Here's how the part is built. I have some questions about the finished solid (model axes, mm). A direction names the side the tool comes from. Coordinates: 2 decimals unless noted, no trailing zeros. Write each loop counter-clockwise with the first axis right and the second up, starting at its lowest first coordinate (ties: lowest second). Pieces come first, ordered by that corner, then holes.
(1) Which directions (+Z, -Z, +X, -X, +Y, -Y) give clear straight access to the entire face, cutting with the end or side of a thin tool? Please do faces 4 (the flat face through (30, 29, 11)), 5 (the flat face through (-30, 29, 11)), 6 (the flat face through (40, 17, 0)), 7 (the cylindrical face through (23.846, 22.675, -7.509)).
(2) Imagine slicing it at B-B, the plane y = 24. List the corners of the cut face in (x, z) for me, plus the area to 3 significant figures.
(3) Please list where these lines run through material, in increasing order: probe 1 along X at (y, z) = (27, 0); probe 2 along X at (y, z) = (4.5, 0); probe 3 along Z at (x, y) = (35.5, 30.5).
(4) Imagine slicing it at C-C, the plane x = 6. List the corners of the cut face in (y, z) for me.
(5) Imagine slicing it at A-A, the plane z = 0. List the corners of the cut face in (x, y) for me, plus the area to 3 significant figures.
(6) For pin 1 Ø10 at (x, y) = (-10.5, 8) entering from -Z; pin 2 Ø3 at (x, y) = (13, 24) entering from +Z; pin 3 Ø3 at (y, z) = (16.5, 26) entering from +X, each with a flat end and sliding along its axis, tell me the tip position at first contact or that it passes through.
(7) Imagine slicing it at D-D, the plane y = 7.5. List the corners of the cut face in (x, z) for me.
(8) Thinking about a two-plate mould opening in X: for faces 1 (the cylindrical face through (-0.37, 5.07, 10.65)), 2 (the flat face through (-30, 29, -12)), 3 (the flat face through (30, 6, 11)), which applies, released by +X, released by -X, zero draft, split by the parting line, or undercut?
```python
from build123d import *

# Parameters (mm, degrees)
BOSS_EXTRUDE1_DEPTH = 35
SKETCH2_R           = 2.8
CUT_EXTRUDE1_DEPTH  = 10
CUT_EXTRUDE2_START  = -80
SKETCH2_2_R         = 2.8
CUT_EXTRUDE2_DEPTH  = 10
SKETCH3_R           = 1.69
SKETCH3_R_2         = 2.25
CUT_EXTRUDE3_DEPTH  = 36
SKETCH4_R           = 25
CUT_EXTRUDE4_DEPTH  = 25


with BuildPart() as part:
    # Sketch1 → Boss-Extrude1 (new body)
    with BuildSketch(Plane(origin=(0, 0, 0), x_dir=(1, 0, 0), z_dir=(0, 1, 0))):
        with BuildLine():
            Line((-40, 17.5), (-40, -17.5))
            ThreePointArc((-40, -17.5), (0, -43.660622991), (40, -17.5))
            Line((40, -17.5), (40, 17.5))
            ThreePointArc((40, 17.5), (0, 43.660622991), (-40, 17.5))
        make_face()
    extrude(amount=BOSS_EXTRUDE1_DEPTH)

    # Sketch2 → Cut-Extrude1 (cut)
    with BuildSketch(Plane.ZY.offset(40)):
        with Locations((-11.5, 29)):
            Circle(SKETCH2_R)
        with Locations((11.5, 29)):
            Circle(SKETCH2_R)
        with Locations((-11.5, 6)):
            Circle(SKETCH2_R)
        with Locations((11.5, 6)):
            Circle(SKETCH2_R)
    extrude(amount=-CUT_EXTRUDE1_DEPTH, mode=Mode.SUBTRACT)

    # Sketch2<2> → Cut-Extrude2 (cut)
    with BuildSketch(Plane.ZY.offset(40).offset(CUT_EXTRUDE2_START)):
        with Locations((-11.5, 29)):
            Circle(SKETCH2_2_R)
        with Locations((11.5, 29)):
            Circle(SKETCH2_2_R)
        with Locations((-11.5, 6)):
            Circle(SKETCH2_2_R)
        with Locations((11.5, 6)):
            Circle(SKETCH2_2_R)
    extrude(amount=CUT_EXTRUDE2_DEPTH, mode=Mode.SUBTRACT)

    # Sketch3 → Cut-Extrude3 (cut, through all)
    with BuildSketch(Plane(origin=(0, 35, 0), x_dir=(1, 0, 0), z_dir=(0, 1, 0))):
        with Locations((0, 9)):
            Circle(SKETCH3_R)
        with Locations((6, 0)):
            Circle(SKETCH3_R)
        with Locations((0, -9)):
            Circle(SKETCH3_R)
        with Locations((-6, 0)):
            Circle(SKETCH3_R)
        Circle(SKETCH3_R_2)
    extrude(amount=-CUT_EXTRUDE3_DEPTH, mode=Mode.SUBTRACT)

    # Sketch4 → Cut-Extrude4 (cut)
    with BuildSketch(Plane(origin=(0, 35, 0), x_dir=(1, 0, 0), z_dir=(0, 1, 0))):
        Circle(SKETCH4_R)
    extrude(amount=-CUT_EXTRUDE4_DEPTH, mode=Mode.SUBTRACT)


solid = part.part
```
Recorded:
1. face 4: +X
1. face 5: -X
1. face 6: +Z, -Z, +X, +Y, -Y
1. face 7: +Y
2. outline: (-40, -17.5) arc R43.66 ccw to (40, -17.5) - (40, 17.5) arc R43.66 ccw to (-40, 17.5) - close; hole circle Ø50 at (0, 0)
2. area: 3,850 mm2
3. probe 1: x = -40 to -25, 25 to 40
3. probe 2: x = -40 to -7.69, -4.31 to -2.25, 2.25 to 4.31, 7.69 to 40
3. probe 3: z = -25.42 to -13.86, -9.14 to 9.14, 13.86 to 25.42
4. outline: (0, -43.25) - (35, -43.25) - (35, -24.27) - (10, -24.27) - (10, -1.69) - (0, -1.69) - close; (0, 1.69) - (10, 1.69) - (10, 24.27) - (35, 24.27) - (35, 43.25) - (0, 43.25) - close
5. outline: (-40, 0) - (-7.69, 0) - (-7.69, 10) - (-25, 10) - (-25, 35) - (-40, 35) - close; (-4.31, 0) - (-2.25, 0) - (-2.25, 10) - (-4.31, 10) - close; (2.25, 0) - (4.31, 0) - (4.31, 10) - (2.25, 10) - close; (7.69, 0) - (40, 0) - (40, 35) - (25, 35) - (25, 10) - (7.69, 10) - close
5. area: 1,440 mm2
6. pin 1: stops at z = -43.31
6. pin 2: stops at z = 42.12
6. pin 3: stops at x = 36.14
7. outline: (-40, -17.5) arc R43.66 ccw to (40, -17.5) - (40, -13.86) - (30, -13.86) - (30, -9.14) - (40, -9.14) - (40, 9.14) - (30, 9.14) - (30, 13.86) - (40, 13.86) - (40, 17.5) arc R43.66 ccw to (-40, 17.5) - (-40, 13.86) - (-30, 13.86) - (-30, 9.14) - (-40, 9.14) - (-40, -9.14) - (-30, -9.14) - (-30, -13.86) - (-40, -13.86) - close; hole circle Ø3.38 at (-6, 0); hole circle Ø4.5 at (0, 0); hole circle Ø3.38 at (0, -9); hole circle Ø3.38 at (0, 9); hole circle Ø3.38 at (6, 0)
8. face 1: undercut
8. face 2: released by -X
8. face 3: released by +X
